from build123d import *

# Parameters (mm, degrees)
F2_W     = 7.75
F2_H     = 1.55
F3_DEPTH = 1.72
F4_SIZE  = 0.75


with BuildPart() as f1:
    # F0 (on Front) → F1 (revolve)
    with BuildSketch(Plane.XZ):
        Polygon((0, 4.15), (0, 0), (5, 0), (7.9, 0), (7.9, 4.15), (7.9, 6.75), (5, 6.75), (5, 4.15), align=None)
    revolve(axis=Axis((0, 0, 2.075), (0, 0, 1)))

    # F2 (on face) → F3 (cut)
    with BuildSketch(Plane(origin=(0, 0, 0), x_dir=(1, 0, 0), z_dir=(0, 0, -1))):
        Rectangle(F2_W, F2_H)
    extrude(amount=-F3_DEPTH, mode=Mode.SUBTRACT)

    # F4
    f4_edges = [f1.edges().sort_by_distance(p)[0] for p in [
        (-5, 0, 6.75),
    ]]
    chamfer(f4_edges, length=F4_SIZE)


solid = f1.part
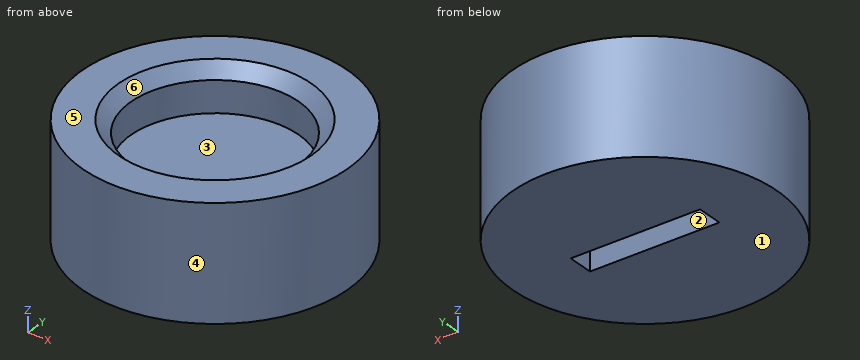
For this review, take the finished solid that the model builds, in its own axes (mm). Face numbers are marked on the shaded views. A direction names the side the tool comes from. Coordinates: 2 decimals unless noted, no trailing zeros. Write each loop counter-clockwise with the first axis right and the second up, starting at its lowest first coordinate (ties: lowest second). Pieces come first, ordered by that corner, then holes. Notation, with made-up numbers: (12.5, 60) -> (17.5, 60) arc R25 ccw to (17.5, 92) -> close; hole circle Ø10 at (19, 88.25). An arc over 180 degrees is marked (long way). Write each question's results on one line, items separated by ' | '. Start each with the question number.
1) Insertion check: pin 1 (0.5 mm diameter, centred on y = -0.5, z = 1, fed in from -X); pin 2 (0.5 mm diameter, centred on x = 0.5, z = 0.5, fed in from +Y); pin 3 (0.8 mm diameter, centred on x = 1, y = 0, fed in from -Z). Each pin has a flat end and moves straight along its axis. Give the tip position at first contact, or say it passes through.
2) Consider section C-C (z = 3). Write out the cut boundary in (x, y), plus the area to 3 significant figures.
3) Consider section B-B (x = 0). Write out the cut boundary in (y, z) (3 decimals).
4) The part is to be moulded in two halves that separate along Y. For the marked faces 4, 5 and 6, say which applies: +Y half, -Y half, draft (parallel to the pull), parting line (faces both ways), or undercut.
5) For the marked faces 1, 2 and 3, list the 3-axis set-ups (+Z, -Z, +X, -X, +Y, -Y) from which the entire face can be reached by the end or side of a thin tool; tool diameter is ignored.
6) Wall thickness on L1, parallel to Y at x = 0, z = 4.85; L2, parallel to Z at x = -4.25, y = 1; L3, parallel to Z at x = 2.5, y = 0: over which ranges is each line inside the solid? List them lowest first. Write a range as [from, to].
7) Consider section D-D (x = 6). Write out the cut boundary in (y, z).
8) Consider section A-A (y = 0). Write out the cut boundary in (x, z) (3 decimals), plus the area to 3 significant figures.
Geometry says:
1) pin 1: x = -7.9 | pin 2: y = 7.9 | pin 3: z = 1.72
2) outline: circle Ø15.8 at (0, 0) | area: 196 mm^2
3) outline: (-7.9, 0) -> (-0.775, 0) -> (-0.775, 1.72) -> (0.775, 1.72) -> (0.775, 0) -> (7.9, 0) -> (7.9, 6.75) -> (5.75, 6.75) -> (5, 6) -> (5, 4.15) -> (-5, 4.15) -> (-5, 6) -> (-5.75, 6.75) -> (-7.9, 6.75) -> close
4) face 4: parting line | face 5: draft | face 6: undercut
5) face 1: -Z, +X, -X, +Y, -Y | face 2: -Z | face 3: +Z
6) L1: [-7.9, -5], [5, 7.9] | L2: [0, 4.15] | L3: [1.72, 4.15]
7) outline: (-5.14, 0) -> (5.14, 0) -> (5.14, 6.75) -> (-5.14, 6.75) -> close
8) outline: (-7.9, 0) -> (-3.875, 0) -> (-3.875, 1.72) -> (3.875, 1.72) -> (3.875, 0) -> (7.9, 0) -> (7.9, 6.75) -> (5.75, 6.75) -> (5, 6) -> (5, 4.15) -> (-5, 4.15) -> (-5, 6) -> (-5.75, 6.75) -> (-7.9, 6.75) -> close | area: 66.8 mm^2
